Source: CAD feature listing. Evaluate the final solid. Frame: model axes, mm. Give positions to 0.01 mm unless a question says otherwise; leave off trailing zeros. Order: outer loops, then holes, each group sorted by start corner. A loop starts at its lowest first (then second) coordinate and runs counter-clockwise, first axis right, second up. Notation, with made-up numbers: M 37,49.5 L 59,49.5 A10 ccw 59,54.5 Z; hole C 63.25,53 d6. An arc over 180 degrees is marked long. Answer in a Markdown table with one row per item. Add a question column.
(1) Section query A-A, the plane z = 37.15. Return loops of the section in (x, y), plus the area to 3 significant figures.
(2) Material intervals for line 1 along Z through (x, y) = (70, 2.1); line 2 along X through (y, z) = (1.2, 43); line 3 along Z through (x, y) = (-31, 0.4), sorted ascending.
(3) Mould query, pull axis Z, two halves, no side actions, for faces 1 (the face through (-68.468, 1.521, 34.747)), 2 (the face through (-2, 3, -2)). Classes: pulls with the +Z half, pulls with the -Z half, needs draft (parallel to the pull), parting line crosses it, or undercut.
(4) Pin query (flat end, axial travel): P1, Ø3, axis at x = -30, z = 0, coming from the +Y side; P2, Ø4, axis at x = 30, z = 0, coming from the -Y side. Return the tip coordinate at first contact, or that it passes through.
from build123d import *

# Parameters (mm, degrees)
SKETCH1_W           = 220
SKETCH1_H           = 220
BOSS_EXTRUDE1_DEPTH = 3
SKETCH3_R           = 2.85
CUT_EXTRUDE5_DEPTH  = 4
SKETCH2_R           = 1.7526
CUT_EXTRUDE6_DEPTH  = 4


with BuildPart() as part:
    # Sketch1 → Boss-Extrude1 (new body)
    with BuildSketch(Plane(origin=(0, 0, 0), x_dir=(1, 0, 0), z_dir=(0, 1, 0))):
        Rectangle(SKETCH1_W, SKETCH1_H)
    extrude(amount=BOSS_EXTRUDE1_DEPTH)

    # Sketch3 → Cut-Extrude5 (cut, through all)
    with BuildSketch(Plane(origin=(0, 3, 0), x_dir=(1, 0, 0), z_dir=(0, 1, 0))):
        with Locations((70, -37.15)):
            Circle(SKETCH3_R)
        with Locations((-70, -37.15)):
            Circle(SKETCH3_R)
        with Locations((-70, 37.15)):
            Circle(SKETCH3_R)
        with Locations((70, 37.15)):
            Circle(SKETCH3_R)
    extrude(amount=-CUT_EXTRUDE5_DEPTH, mode=Mode.SUBTRACT)

    # Sketch2 → Cut-Extrude6 (cut, through all)
    with BuildSketch(Plane(origin=(0, 3, 0), x_dir=(1, 0, 0), z_dir=(0, 1, 0))):
        with Locations((-73, 103)):
            Circle(SKETCH2_R)
        with Locations((0, 103)):
            Circle(SKETCH2_R)
        with Locations((-30, 73)):
            Circle(SKETCH2_R)
        with Locations((-103, 73)):
            Circle(SKETCH2_R)
        with Locations((-43, 73)):
            Circle(SKETCH2_R)
        with Locations((0, 43)):
            Circle(SKETCH2_R)
        with Locations((30, 73)):
            Circle(SKETCH2_R)
        with Locations((73, 103)):
            Circle(SKETCH2_R)
        with Locations((43, 73)):
            Circle(SKETCH2_R)
        with Locations((-73, 43)):
            Circle(SKETCH2_R)
        with Locations((73, 43)):
            Circle(SKETCH2_R)
        with Locations((103, 73)):
            Circle(SKETCH2_R)
        with Locations((0, 30)):
            Circle(SKETCH2_R)
        with Locations((-30, 0)):
            Circle(SKETCH2_R)
        with Locations((0, -30)):
            Circle(SKETCH2_R)
        with Locations((30, 0)):
            Circle(SKETCH2_R)
        with Locations((73, 30)):
            Circle(SKETCH2_R)
        with Locations((43, 0)):
            Circle(SKETCH2_R)
        with Locations((73, -30)):
            Circle(SKETCH2_R)
        with Locations((103, 0)):
            Circle(SKETCH2_R)
        with Locations((0, -43)):
            Circle(SKETCH2_R)
        with Locations((-30, -73)):
            Circle(SKETCH2_R)
        with Locations((0, -103)):
            Circle(SKETCH2_R)
        with Locations((30, -73)):
            Circle(SKETCH2_R)
        with Locations((73, -43)):
            Circle(SKETCH2_R)
        with Locations((43, -73)):
            Circle(SKETCH2_R)
        with Locations((73, -103)):
            Circle(SKETCH2_R)
        with Locations((103, -73)):
            Circle(SKETCH2_R)
        with Locations((-73, 30)):
            Circle(SKETCH2_R)
        with Locations((-103, 0)):
            Circle(SKETCH2_R)
        with Locations((-73, -30)):
            Circle(SKETCH2_R)
        with Locations((-43, 0)):
            Circle(SKETCH2_R)
        with Locations((-73, -43)):
            Circle(SKETCH2_R)
        with Locations((-103, -73)):
            Circle(SKETCH2_R)
        with Locations((-73, -103)):
            Circle(SKETCH2_R)
        with Locations((-43, -73)):
            Circle(SKETCH2_R)
    extrude(amount=-CUT_EXTRUDE6_DEPTH, mode=Mode.SUBTRACT)


solid = part.part
Values follow:
| question | item | result |
|---|---|---|
| 1 | outline | M -110,0 L -72.85,0 L -72.85,3 L -110,3 Z; M -67.15,0 L 67.15,0 L 67.15,3 L -67.15,3 Z; M 72.85,0 L 110,0 L 110,3 L 72.85,3 Z |
| 1 | area | 626 mm² |
| 2 | line 1 | z = -110 to -40, -34.3 to 34.3, 40 to 110 |
| 2 | line 2 | x = -110 to -74.75, -71.25 to -1.75, 1.75 to 71.25, 74.75 to 110 |
| 2 | line 3 | z = -110 to -74.44, -71.56 to -1.44, 1.44 to 71.56, 74.44 to 110 |
| 3 | face 1 | undercut |
| 3 | face 2 | needs draft |
| 4 | P1 | passes through |
| 4 | P2 | stops at y = 0 |
